```python
from build123d import *

# Parameters (mm, degrees)
F0_W     = 25.4
F0_H     = 25.4
F0_R     = 6.35
F1_DEPTH = 63.5
F2_R     = 3.175
F3_DEPTH = 25.401


with BuildPart() as f1:
    # F0 (on Top) → F1 (new body)
    with BuildSketch(Plane.XY):
        Rectangle(F0_W, F0_H)
        Circle(F0_R, mode=Mode.SUBTRACT)
    extrude(amount=F1_DEPTH)

    # F2 (on face) → F3 (cut, through all)
    with BuildSketch(Plane.XZ.offset(12.7)):
        with Locations((0, 31.75)):
            Circle(F2_R)
    extrude(amount=-F3_DEPTH, mode=Mode.SUBTRACT)


solid = f1.part
```
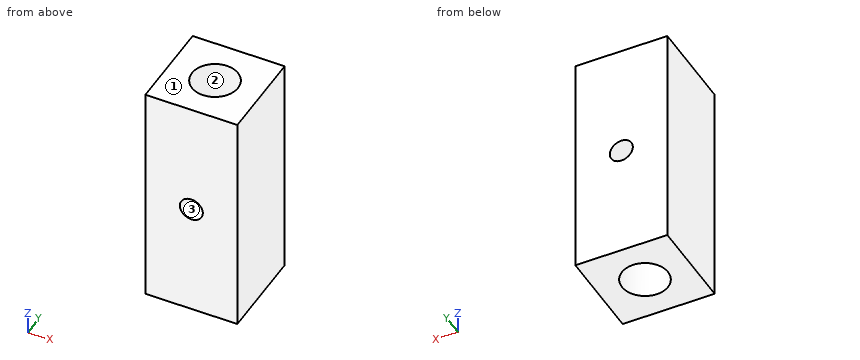
For this review, take the finished solid that the model builds, in its own axes (mm). Face numbers are marked on the shaded views. Coordinates: 2 decimals unless noted, no trailing zeros. Write each loop counter-clockwise with the first axis right and the second up, starting at its lowest first coordinate (ties: lowest second). Pieces come first, ordered by that corner, then holes. Notation, with made-up numbers: (72, 15.25) - (124, 15.25) arc R14 ccw to (124, 32.25) - close; hole circle Ø4 at (57, -27.5). An arc over 180 degrees is marked (long way). Answer in a Markdown table with one row per item. Add a question column.
Q1. For probe 1 along X at (y, z) = (-8.5, 31.75) (3 decimals); probe 2 along Y at (x, z) = (0, 37.5); probe 3 along Z at (x, y) = (0, -8) (3 decimals), list the stretches that pass through material, from the lowest coordinate up.
Q2. We need section B-B, the plane x = 0. State the section outline as (y, z) points (3 decimals).
Q3. We need section C-C, the plane z = 6. State the section outline as (x, y) points, and give its area (3 significant figures).
Q4. We need section D-D, the plane z = 31.75. State the section outline as (x, y) points (3 decimals).
Q5. We need section A-A, the plane y = 0. State the section outline as (x, z) points.
Q6. Draft analysis for pull direction Z (two halves, no side actions). For the marked faces 1, 2 and 3, state which applies: +Z half, -Z half, draft (parallel to the pull), parting line (faces both ways), or undercut.
Answer list:
| question | item | result |
|---|---|---|
| 1 | probe 1 | x = -12.7 to -3.175, 3.175 to 12.7 |
| 1 | probe 2 | y = -12.7 to -6.35, 6.35 to 12.7 |
| 1 | probe 3 | z = 0 to 28.575, 34.925 to 63.5 |
| 2 | outline | (-12.7, 0) - (-6.35, 0) - (-6.35, 28.575) - (-12.7, 28.575) - close; (-12.7, 34.925) - (-6.35, 34.925) - (-6.35, 63.5) - (-12.7, 63.5) - close; (6.35, 0) - (12.7, 0) - (12.7, 28.575) - (6.35, 28.575) - close; (6.35, 34.925) - (12.7, 34.925) - (12.7, 63.5) - (6.35, 63.5) - close |
| 3 | outline | (-12.7, -12.7) - (12.7, -12.7) - (12.7, 12.7) - (-12.7, 12.7) - close; hole circle Ø12.7 at (0, 0) |
| 3 | area | 518 mm2 |
| 4 | outline | (-12.7, -12.7) - (-3.175, -12.7) - (-3.175, -5.499) arc R6.35 cw to (-3.175, 5.499) - (-3.175, 12.7) - (-12.7, 12.7) - close; (3.175, -12.7) - (12.7, -12.7) - (12.7, 12.7) - (3.175, 12.7) - (3.175, 5.499) arc R6.35 cw to (3.175, -5.499) - close |
| 5 | outline | (-12.7, 0) - (-6.35, 0) - (-6.35, 63.5) - (-12.7, 63.5) - close; (6.35, 0) - (12.7, 0) - (12.7, 63.5) - (6.35, 63.5) - close |
| 6 | face 1 | +Z half |
| 6 | face 2 | draft |
| 6 | face 3 | undercut |
